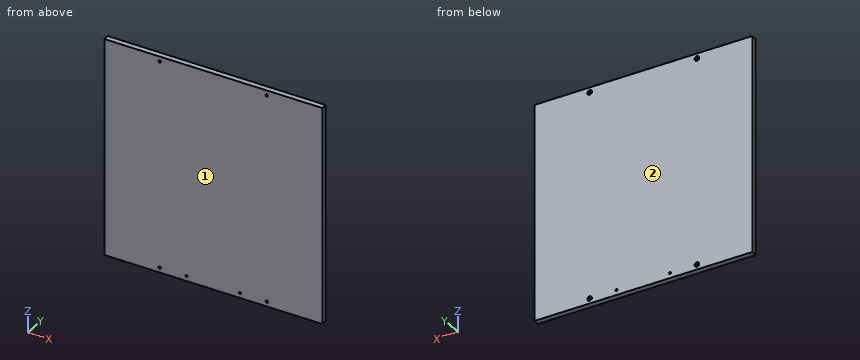
from build123d import *

# Parameters (mm, degrees)
SKETCH_1_W                     = 305
SKETCH_1_H                     = 305
EXTRUDE_1_DEPTH                = 8
HOLE_WIZARD_M1_6_1_D           = 3.4
HOLE_WIZARD_M1_6_1_CBORE_D     = 6.5
HOLE_WIZARD_M1_6_1_CBORE_DEPTH = 3
HOLE_WIZARD_M3_1_D             = 3


with BuildPart() as part:
    # 草图1 → 凸台-拉伸1 (new body)
    with BuildSketch(Plane(origin=(0, 0, 0), x_dir=(1, 0, 0), z_dir=(0, 1, 0))):
        Rectangle(SKETCH_1_W, SKETCH_1_H)
    extrude(amount=EXTRUDE_1_DEPTH)

    # M1.6 六角头螺栓的柱形沉头孔1 (through all)
    with Locations(Plane(origin=(0, 8, 0), x_dir=(1, 0, 0), z_dir=(0, 1, 0))):
        with Locations((-75, 145.5), (75, 145.5), (75, -145.5), (-75, -145.5)):
            CounterBoreHole(HOLE_WIZARD_M1_6_1_D / 2, HOLE_WIZARD_M1_6_1_CBORE_D / 2, HOLE_WIZARD_M1_6_1_CBORE_DEPTH)

    # M3 螺纹孔1 (through all)
    with Locations(Plane(origin=(-37.5, 8, -145.5), x_dir=(0, 0, 1), z_dir=(0, 1, 0))):
        with Locations((0, 0), (0, 75)):
            Hole(HOLE_WIZARD_M3_1_D / 2)


solid = part.part
Verification items for the finished model (mm, model axes). Face numbers are marked on the shaded views. Give positions to 0.01 mm unless a question says otherwise; leave off trailing zeros. Use CSV: the item, a comma, the result in double quotes.
1) Release check for a two-part mould opening along Y. For the marked faces 1 and 2 record: released by +Y, released by -Y, zero draft, split by the parting line, or undercut.
Final values:
face 1,"released by -Y"
face 2,"released by +Y"
2) Material ranges on line 1 along X through (y, z) = (5.9, 145.5); line 2 along Z through (x, y) = (-75, 3.35); line 3 along X through (y, z) = (2.45, -145.5), recorded low to high.
Final values:
line 1,"-152.5 to -78.25, -71.75 to 71.75, 78.25 to 152.5"
line 2,"-152.5 to -147.2, -143.8 to 143.8, 147.2 to 152.5"
line 3,"-152.5 to -76.7, -73.3 to -39, -36 to 36, 39 to 73.3, 76.7 to 152.5"
3) Go/stop test with flat-tipped pins: pin 1 Ø2.5 at (x, z) = (75, -145.5) entering from +Y; pin 2 Ø6 at (x, z) = (-75, -145.5) entering from +Y. Record where each tip stops, or that it passes through.
Final values:
pin 1,"through"
pin 2,"y = 5"
